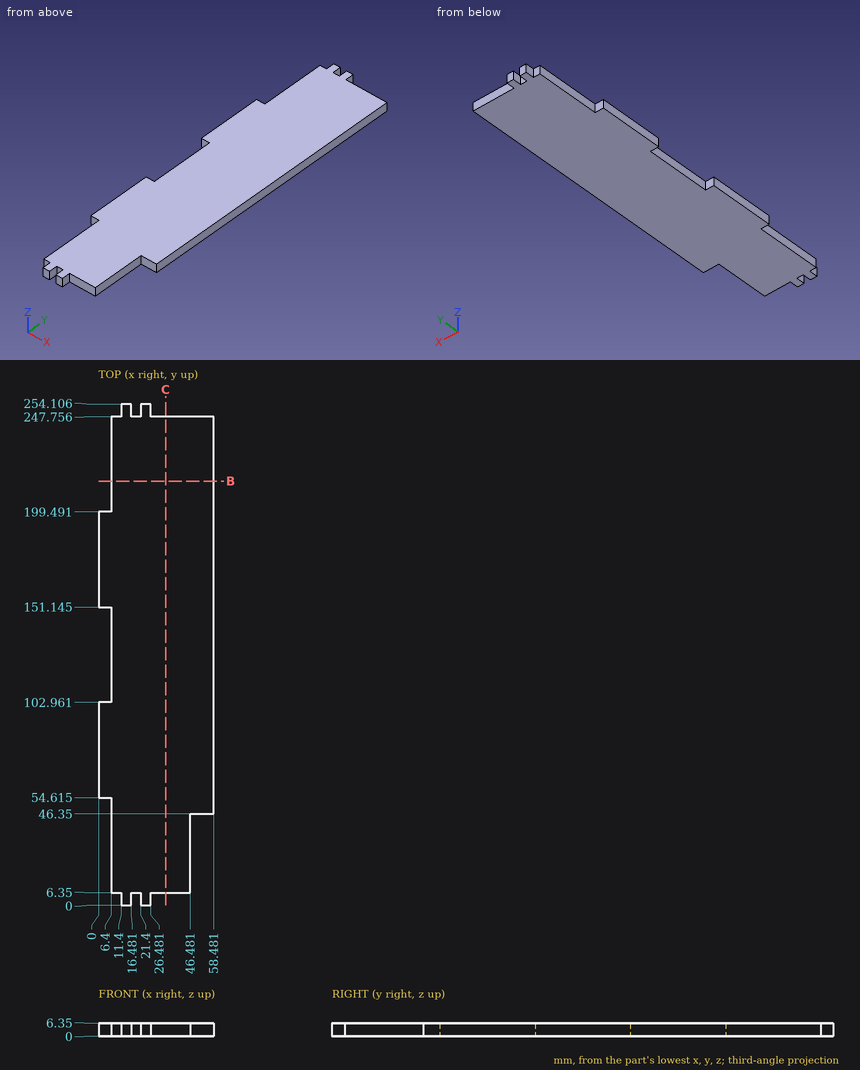
Verification items for this drawing (mm, ordinates from the low corner). Coordinates: 2 decimals unless noted, no trailing zeros. Write each loop counter-clockwise with the first axis right and the second up, starting at its lowest first coordinate (ties: lowest second). Pieces come first, ordered by that corner, then holes. Notation, with made-up numbers: M 38,43 L 57,43 A9 ccw 57,52 Z; hole C 19,48.5 d1. An arc over 180 degrees is marked long. One line per item, written item: value. Start each with the question number.
(1) Sectioned sample at C-C, the plane x = 34. Enter the section's corners in (y, z).
(2) Depth check by flat-ended pin: pin 1 (3 mm diameter, centred on y = 2.5, z = 4.5, fed in from -X); pin 2 (1.5 mm diameter, centred on x = 33, z = 5.5, fed in from +Y); pin 3 (1 mm diameter, centred on x = 20, z = 5, fed in from -Y). Enter the tip coordinate at first touch or a pass-through.
(3) Sectioned sample at B-B, the plane y = 215. Enter the section's corners in (x, z).
(4) Scan lines: line 1 along Y through (x, z) = (6, 5) (1 decimal); line 2 along Y through (x, z) = (48.5, 4.25); line 3 along X through (y, z) = (214.5, 2). Record each from-to range of solid material in increasing order. Write a range as [from, to].
Filled sheet:
1. outline: M 6.35,0 L 247.76,0 L 247.76,6.35 L 6.35,6.35 Z
2. pin 1: x = 11.4
2. pin 2: y = 247.76
2. pin 3: y = 6.35
3. outline: M 6.4,0 L 58.48,0 L 58.48,6.35 L 6.4,6.35 Z
4. line 1: [54.6, 103], [151.1, 199.5]
4. line 2: [46.35, 247.76]
4. line 3: [6.4, 58.48]
